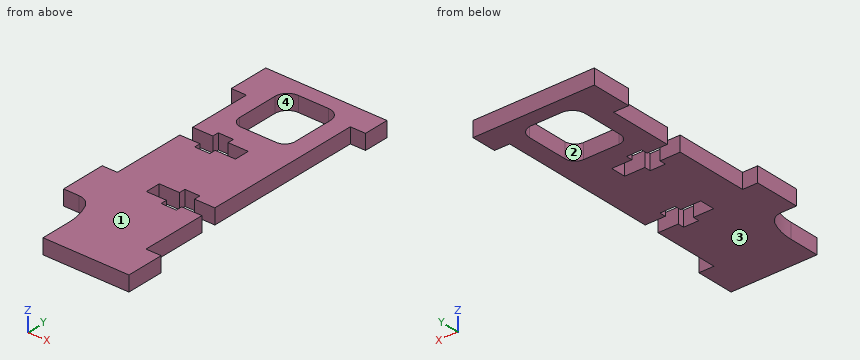
```python
from build123d import *

# Parameters (mm, degrees)
BOSS_EXTRUDE1_DEPTH = 3


with BuildPart() as part:
    # Model → Boss-Extrude1 (new body)
    with BuildSketch(Plane.XY):
        with BuildLine():
            Line((71, 68), (71, 63))
            Line((71, 63), (68, 63))
            Line((68, 63), (68, 31.5))
            Line((68, 31.5), (64, 31.5))
            Line((64, 31.5), (64, 32.75))
            Line((64, 32.75), (61, 32.75))
            Line((61, 32.75), (61, 31.5))
            Line((61, 31.5), (57, 31.5))
            Line((57, 31.5), (57, 28.5))
            Line((57, 28.5), (61, 28.5))
            Line((61, 28.5), (61, 27.25))
            Line((61, 27.25), (64, 27.25))
            Line((64, 27.25), (64, 28.5))
            Line((64, 28.5), (68, 28.5))
            Line((68, 28.5), (68, 15.5))
            Line((68, 15.5), (71, 15.5))
            Line((71, 15.5), (71, 8))
            Line((71, 8), (54, 8))
            Line((54, 8), (54, 14))
            ThreePointArc((54, 14), (53.719770148, 16.588625278), (52.861029282, 19.046688281))
            ThreePointArc((52.861029282, 19.046688281), (51.73197083, 20.444193402), (50.0235, 21))
            Line((50.0235, 21), (47, 21))
            Line((47, 21), (47, 30))
            Line((47, 30), (50, 30))
            Line((50, 30), (50, 44.5))
            Line((50, 44.5), (54, 44.5))
            Line((54, 44.5), (54, 43.25))
            Line((54, 43.25), (57, 43.25))
            Line((57, 43.25), (57, 44.5))
            Line((57, 44.5), (61, 44.5))
            Line((61, 44.5), (61, 47.5))
            Line((61, 47.5), (57, 47.5))
            Line((57, 47.5), (57, 48.75))
            Line((57, 48.75), (54, 48.75))
            Line((54, 48.75), (54, 47.5))
            Line((54, 47.5), (50, 47.5))
            Line((50, 47.5), (50, 60))
            Line((50, 60), (47, 60))
            Line((47, 60), (47, 68))
            Line((47, 68), (71, 68))
        make_face()
        with BuildLine():
            Line((56, 65), (62, 65))
            ThreePointArc((62, 65), (63.76778125, 64.26778125), (64.5, 62.5))
            Line((64.5, 62.5), (64.5, 54.25))
            ThreePointArc((64.5, 54.25), (63.914214645, 52.835814644), (62.5, 52.2501))
            Line((62.5, 52.2501), (55.5, 52.2501))
            ThreePointArc((55.5, 52.2501), (54.085735358, 52.835764643), (53.5, 54.25))
            Line((53.5, 54.25), (53.5, 62.5))
            ThreePointArc((53.5, 62.5), (54.2322, 64.2678), (56, 65))
        make_face(mode=Mode.SUBTRACT)
    extrude(amount=BOSS_EXTRUDE1_DEPTH)


solid = part.part
```
Geometry check sheet. Reference: the model listing, model coordinates, mm. Face numbers are marked on the shaded views. A direction names the side the tool comes from. Round coordinates to 2 decimals unless told otherwise and drop trailing zeros. Loops run counter-clockwise (first coordinate to the right, second up) from the corner with the lowest first, then second, coordinate; pieces in that order, holes last. Notation, with made-up numbers: M 46,65.25 L 101,65.25 A24 cw 101,78.25 Z; hole C 82,-39 d6. An arc over 180 degrees is marked long. Return JSON: item names as keys, results as strings. Group by question number.
(1) Mould release check, pull along X, two halves, no side actions. Record for the marked faces 3 and 4: pulls with the +X half, pulls with the -X half, needs draft (parallel to the pull), parting line crosses it, or undercut.
(2) Section check B-B, the plane y = 57.5. Enter the section's corners in (x, z).
(3) Set-up check for the marked faces 1 and 2: record each of +Z, -Z, +X, -X, +Y, -Y from which the full face is reachable in a straight line by a thin tool's end or side.
(4) Section check A-A, the plane x = 67. Enter the section's corners in (y, z).
(5) Scan lines: line 1 along Y through (x, z) = (60.5, 2.75); line 2 along Y through (x, z) = (61.75, 2.6); line 3 along Y through (x, z) = (67.75, 1.05). Record each from-to range of solid material in increasing order. Write a range as [from, to].
(6) Go/stop test with flat-tipped pins: pin 1 (1.5 mm diameter, centred on y = 46, z = 1.5, fed in from -X); pin 2 (1 mm diameter, centred on y = 48.5, z = 1.5, fed in from +X); pin 3 (0.6 mm diameter, centred on y = 43.5, z = 1, fed in from -X). Record where each tip stops, or that it passes through.
Data:
{
 "1": {"face 3": "needs draft", "face 4": "undercut"},
 "2": {"outline": "M 50,0 L 53.5,0 L 53.5,3 L 50,3 Z; M 64.5,0 L 68,0 L 68,3 L 64.5,3 Z"},
 "3": {"face 1": "+Z, +X, -X, +Y, -Y", "face 2": "+Z, -Z"},
 "4": {"outline": "M 8,0 L 28.5,0 L 28.5,3 L 8,3 Z; M 31.5,0 L 68,0 L 68,3 L 31.5,3 Z"},
 "5": {"line 1": "[8, 28.5], [31.5, 44.5], [47.5, 52.25], [65, 68]", "line 2": "[8, 27.25], [32.75, 52.25], [65, 68]", "line 3": "[8, 28.5], [31.5, 68]"},
 "6": {"pin 1": "x = 61", "pin 2": "x = 68", "pin 3": "x = 50"}
}
